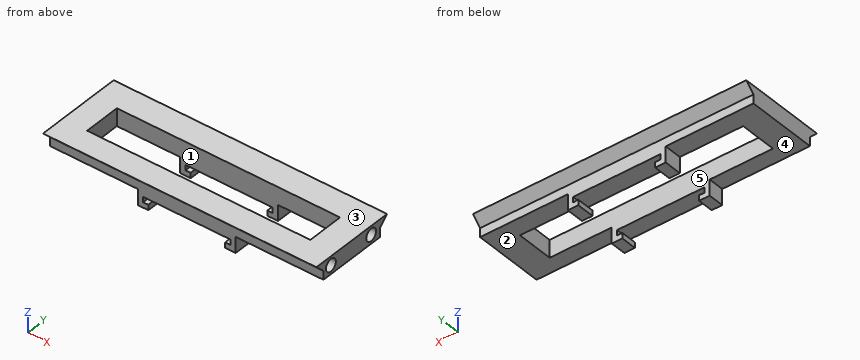
```python
from build123d import *

# Parameters (mm, degrees)
BOSS_EXTRUDE1_DEPTH = 40
SKETCH2_W           = 127.211228058
SKETCH2_H           = 21.064469041
CUT_EXTRUDE1_DEPTH  = 60
BOSS_EXTRUDE2_DEPTH = 155.8
SKETCH4_R           = 3.5
CUT_EXTRUDE2_DEPTH  = 150


with BuildPart() as part:
    # Sketch1 → Boss-Extrude1 (new body)
    with BuildSketch(Plane(origin=(0, 0, 0), x_dir=(1, 0, 0), z_dir=(0, 1, 0))):
        Polygon((-60.768130494, -10.644024468), (-63.768130494, -10.644024468), (-63.768130494, -19.644024468), (-113.768130494, -19.644024468), (-113.768130494, -29.644024468), (42.031869506, -29.644024468), (42.031869506, -19.644024468), (-7.968130494, -19.644024468), (-7.968130494, -10.644024468), (-10.968130494, -10.644024468), (-13.968130494, -10.644024468), (-13.968130494, -13.726650188), (-10.968130494, -13.644024468), (-10.968130494, -16.726650188), (-13.968130494, -16.726650188), (-57.768130494, -16.726650188), (-60.768130494, -16.726650188), (-60.768130494, -13.644024468), (-57.768130494, -13.726650188), (-57.768130494, -10.644024468), align=None)
    extrude(amount=BOSS_EXTRUDE1_DEPTH)

    # Sketch2 → Cut-Extrude1 (cut)
    with BuildSketch(Plane.XY.offset(29.644024468)):
        with Locations((-36.201542798, 19.418495801)):
            Rectangle(SKETCH2_W, SKETCH2_H)
    extrude(amount=-CUT_EXTRUDE1_DEPTH, mode=Mode.SUBTRACT)

    # Sketch3 → Boss-Extrude2 (add)
    with BuildSketch(Plane(origin=(42.031869506, 0, 0), x_dir=(0, 0, -1), z_dir=(1, 0, 0))):
        Polygon((-29.644024468, 40), (-24.644024468, 40), (-29.644024468, 45), align=None)
        Polygon((-29.644024468, 0), (-29.644024468, -5), (-24.644024468, 0), align=None)
    extrude(amount=-BOSS_EXTRUDE2_DEPTH)

    # Sketch4 → Cut-Extrude2 (cut)
    with BuildSketch(Plane(origin=(42.031869506, 0, 0), x_dir=(0, 0, -1), z_dir=(1, 0, 0))):
        with Locations((-24.644024468, 33.806203399)):
            Circle(SKETCH4_R)
        with Locations((-24.644024468, 5.303574021)):
            Circle(SKETCH4_R)
    extrude(amount=-CUT_EXTRUDE2_DEPTH, mode=Mode.SUBTRACT)


solid = part.part
```
Design review of the part built by this model. Coordinates are the model's own, in mm. Face numbers are marked on the shaded views. A direction names the side the tool comes from. Coordinates: 2 decimals unless noted, no trailing zeros. Order: outer loops, then holes, each group sorted by start corner. A loop starts at its lowest first (then second) coordinate and runs counter-clockwise, first axis right, second up.
1) Take a section at D-D, the plane y = 42. Give the boundary of the cut face in (x, z), and give its area (3 significant figures).
2) Take a section at C-C, the plane x = -74.5. Give the boundary of the cut face in (y, z).
3) Clearance check with flat-ended pins moving along their axes: pin 1 (5 mm diameter, centred on x = -60.5, z = 14.5, fed in from -Y); pin 2 (9.5 mm diameter, centred on x = -8, z = 22, fed in from -Y); pin 3 (1.5 mm diameter, centred on y = 5.5, z = 15, fed in from +X); pin 4 (10 mm diameter, centred on x = -72.5, y = 24, fed in from +Z). State where each tip first meets the part, or that it passes through.
4) Take a section at B-B, the plane x = -55.5. Give the boundary of the cut face in (y, z), and give its area (3 significant figures).
5) Take a section at A-A, the plane y = 11. Give the boundary of the cut face in (x, z).
6) For the marked faces 1, 2 and 3, list the 3-axis set-ups (+Z, -Z, +X, -X, +Y, -Y) from which the entire face can be reached by the end or side of a thin tool; tool diameter is ignored.
7) Mouldability with a two-part tool opening along X and no side actions: class the marked faces 4 and 5 as +X half, -X half, draft (parallel to the pull), parting line (faces both ways), or undercut.
8) Wall thickness on line 1 along Y through (x, z) = (-82, 20); line 2 along X through (y, z) = (35, 13.25); line 3 along Y through (x, z) = (-66.5, 22.5): over which ranges is each line inside the solid? List them lowest first.
Returned:
1. outline: (-113.77, 26.64) - (42.03, 26.64) - (42.03, 29.64) - (-113.77, 29.64) - close
1. area: 467 mm2
2. outline: (-5, 29.64) - (0, 24.64) - (0, 19.64) - (8.89, 19.64) - (8.89, 29.64) - close; (29.95, 19.64) - (40, 19.64) - (40, 24.64) - (45, 29.64) - (29.95, 29.64) - close; hole circle Ø7 at (5.3, 24.64); hole circle Ø7 at (33.81, 24.64)
3. pin 1: stops at y = 0
3. pin 2: stops at y = -2.11
3. pin 3: stops at x = -7.97
3. pin 4: passes through
4. outline: (-5, 29.64) - (0, 24.64) - (0, 16.73) - (8.89, 16.73) - (8.89, 29.64) - close; (29.95, 16.73) - (40, 16.73) - (40, 24.64) - (45, 29.64) - (29.95, 29.64) - close; hole circle Ø7 at (5.3, 24.64); hole circle Ø7 at (33.81, 24.64)
4. area: 193 mm2
5. outline: (-113.77, 19.64) - (-99.81, 19.64) - (-99.81, 29.64) - (-113.77, 29.64) - close; (27.4, 19.64) - (42.03, 19.64) - (42.03, 29.64) - (27.4, 29.64) - close
6. face 1: +Z, -Z
6. face 2: -Z, +X, +Y, -Y
6. face 3: +Z, +X, -X, +Y, -Y
7. face 4: draft
7. face 5: undercut
8. line 1: y = 0 to 8.89, 29.95 to 40
8. line 2: x = -63.77 to -57.77, -13.97 to -7.97
8. line 3: y = 0 to 2.54, 8.07 to 8.89, 29.95 to 31.04, 36.57 to 40
